For this review, take the finished solid that the model builds, in its own axes (mm). A direction names the side the tool comes from. Coordinates: 2 decimals unless noted, no trailing zeros. Order: outer loops, then holes, each group sorted by start corner. A loop starts at its lowest first (then second) coordinate and runs counter-clockwise, first axis right, second up. Notation, with made-up numbers: M 18,46.5 L 46,46.5 A21 cw 46,58.5 Z; hole C 60,11.5 d10. An arc over 180 degrees is marked long. Use one line per item in the form item = value. Start each with the question number.
```python
from build123d import *

# Parameters (mm, degrees)
SKETCH_1_W           = 200
SKETCH_1_H           = 250
EXTRUDE_1_DEPTH      = 5
CUT_EXTRUDE_1_DEPTH  = 35
CUT_EXTRUDE_2_DEPTH  = 35
CUT_EXTRUDE_5_DEPTH  = 30
CUT_EXTRUDE_6_DEPTH  = 10
SKETCH_9_R           = 1.5
CUT_EXTRUDE_8_DEPTH  = 10
SKETCH_10_R          = 1.5
CUT_EXTRUDE_9_DEPTH  = 10
CUT_EXTRUDE_12_DEPTH = 10
SKETCH_15_R          = 1.5
CUT_EXTRUDE_13_DEPTH = 10
SKETCH_16_R          = 1.5
CUT_EXTRUDE_14_DEPTH = 10
CUT_EXTRUDE_15_DEPTH = 10


with BuildPart() as part:
    # 草图1 → 凸台-拉伸1 (new body)
    with BuildSketch(Plane(origin=(0, 0, 0), x_dir=(1, 0, 0), z_dir=(0, 1, 0))):
        Rectangle(SKETCH_1_W, SKETCH_1_H)
    extrude(amount=EXTRUDE_1_DEPTH)

    # 草图2 → 切除-拉伸1 (cut)
    with BuildSketch(Plane(origin=(0, 5, 0), x_dir=(1, 0, 0), z_dir=(0, 1, 0))):
        Polygon((-100, -115), (-80, -125), (-100, -125), align=None)
    cut_extrude_1 = extrude(amount=-CUT_EXTRUDE_1_DEPTH, mode=Mode.SUBTRACT)

    # 镜向1: 切除-拉伸1 across plane
    add(cut_extrude_1.mirror(Plane(origin=(0, 0, 0), x_dir=(0, 0, 1), z_dir=(1, 0, 0))), mode=Mode.SUBTRACT)

    # 草图3 → 切除-拉伸2 (cut)
    with BuildSketch(Plane(origin=(0, 5, 0), x_dir=(1, 0, 0), z_dir=(0, 1, 0))):
        Polygon((-55, -125), (-50, -120), (0, -120), (0, -125), align=None)
    cut_extrude_2 = extrude(amount=-CUT_EXTRUDE_2_DEPTH, mode=Mode.SUBTRACT)

    # 镜向2: 切除-拉伸2 across plane
    add(cut_extrude_2.mirror(Plane(origin=(0, 0, 0), x_dir=(0, 0, 1), z_dir=(1, 0, 0))), mode=Mode.SUBTRACT)

    # 草图5 → 切除-拉伸5 (cut)
    with BuildSketch(Plane(origin=(0, 0, 0), x_dir=(1, 0, 0), z_dir=(0, 1, 0))):
        Polygon((-30, 125), (-100, 115), (-100, 125), align=None)
    cut_extrude_5 = extrude(amount=CUT_EXTRUDE_5_DEPTH, mode=Mode.SUBTRACT)

    # 镜向3: 切除-拉伸5 across plane
    add(cut_extrude_5.mirror(Plane(origin=(0, 0, 0), x_dir=(0, 0, 1), z_dir=(1, 0, 0))), mode=Mode.SUBTRACT)

    # 草图6 → 切除-拉伸6 (cut)
    with BuildSketch(Plane(origin=(0, 5, 0), x_dir=(1, 0, 0), z_dir=(0, 1, 0))):
        with BuildLine():
            Line((-100, 95), (-90, 95))
            Line((-90, 95), (-90, 105))
            Line((-90, 105), (-80, 105))
            ThreePointArc((-80, 105), (-75.121684822, 101.096376317), (-77.860612309, 95.480816412))
            Line((-77.860612309, 95.480816412), (-100, 85))
            Line((-100, 85), (-100, 95))
        make_face()
    cut_extrude_6 = extrude(amount=-CUT_EXTRUDE_6_DEPTH, mode=Mode.SUBTRACT)

    # 镜向4: 切除-拉伸6 across plane
    add(cut_extrude_6.mirror(Plane(origin=(0, 0, 0), x_dir=(0, 0, 1), z_dir=(1, 0, 0))), mode=Mode.SUBTRACT)

    # 草图9 → 切除-拉伸8 (cut)
    with BuildSketch(Plane(origin=(0, 5, 0), x_dir=(1, 0, 0), z_dir=(0, 1, 0))):
        with Locations((-80, -100)):
            Circle(SKETCH_9_R)
        with Locations((80, -100)):
            Circle(SKETCH_9_R)
    extrude(amount=-CUT_EXTRUDE_8_DEPTH, mode=Mode.SUBTRACT)

    # 草图10 → 切除-拉伸9 (cut)
    with BuildSketch(Plane(origin=(0, 5, 0), x_dir=(1, 0, 0), z_dir=(0, 1, 0))):
        with Locations((-80, 112.806380134)):
            Circle(SKETCH_10_R)
        with Locations((80, 112.806380134)):
            Circle(SKETCH_10_R)
    extrude(amount=-CUT_EXTRUDE_9_DEPTH, mode=Mode.SUBTRACT)

    # 草图14 → 切除-拉伸12 (cut)
    with BuildSketch(Plane(origin=(0, 5, 0), x_dir=(1, 0, 0), z_dir=(0, 1, 0))):
        with BuildLine():
            Line((-100, -85), (-72.5, -85))
            ThreePointArc((-72.5, -85), (-70.732233047, -84.267766953), (-70, -82.5))
            Line((-70, -82.5), (-70, -22.5))
            ThreePointArc((-70, -22.5), (-70.732233047, -20.732233047), (-72.5, -20))
            Line((-72.5, -20), (-100, -20))
            Line((-100, -20), (-100, -85))
        make_face()
        with BuildLine():
            Line((100, -20), (100, -85))
            Line((100, -85), (72.5, -85))
            ThreePointArc((72.5, -85), (70.732233047, -84.267766953), (70, -82.5))
            Line((70, -82.5), (70, -22.5))
            ThreePointArc((70, -22.5), (70.732233047, -20.732233047), (72.5, -20))
            Line((72.5, -20), (100, -20))
        make_face()
    extrude(amount=-CUT_EXTRUDE_12_DEPTH, mode=Mode.SUBTRACT)

    # 草图15 → 切除-拉伸13 (cut)
    with BuildSketch(Plane(origin=(0, 5, 0), x_dir=(1, 0, 0), z_dir=(0, 1, 0))):
        with Locations((-52.53096351, 0)):
            Circle(SKETCH_15_R)
        with Locations((-52.53096351, 86.645023586)):
            Circle(SKETCH_15_R)
        with Locations((52.53096351, 0)):
            Circle(SKETCH_15_R)
        with Locations((52.53096351, 86.645023586)):
            Circle(SKETCH_15_R)
    extrude(amount=-CUT_EXTRUDE_13_DEPTH, mode=Mode.SUBTRACT)

    # 草图16 → 切除-拉伸14 (cut)
    with BuildSketch(Plane.XZ):
        with Locations((60, 62.5)):
            Circle(SKETCH_16_R)
        with Locations((60, 42.5)):
            Circle(SKETCH_16_R)
        with Locations((36, 42.5)):
            Circle(SKETCH_16_R)
        with Locations((36, 62.5)):
            Circle(SKETCH_16_R)
    cut_extrude_14 = extrude(amount=-CUT_EXTRUDE_14_DEPTH, mode=Mode.SUBTRACT)

    # 镜向5: 切除-拉伸14 across plane
    add(cut_extrude_14.mirror(Plane(origin=(0, 0, 0), x_dir=(0, 0, 1), z_dir=(1, 0, 0))), mode=Mode.SUBTRACT)

    # 草图18 → 切除-拉伸15 (cut)
    with BuildSketch(Plane(origin=(0, 5, 0), x_dir=(1, 0, 0), z_dir=(0, 1, 0))):
        with BuildLine():
            Line((-19, -62.5), (19, -62.5))
            ThreePointArc((19, -62.5), (19.707106781, -62.207106781), (20, -61.5))
            Line((20, -61.5), (20, -43.5))
            ThreePointArc((20, -43.5), (19.707106781, -42.792893219), (19, -42.5))
            Line((19, -42.5), (-19, -42.5))
            ThreePointArc((-19, -42.5), (-19.707106781, -42.792893219), (-20, -43.5))
            Line((-20, -43.5), (-20, -61.5))
            ThreePointArc((-20, -61.5), (-19.707106781, -62.207106781), (-19, -62.5))
        make_face()
    extrude(amount=-CUT_EXTRUDE_15_DEPTH, mode=Mode.SUBTRACT)


solid = part.part
```
1. For pin 1 Ø2 at (x, z) = (-18, 45.5) entering from +Y; pin 2 Ø2.5 at (x, y) = (-94.5, 2.5) entering from +Z (3 decimals); pin 3 Ø2.5 at (y, z) = (2, 46) entering from -X; pin 4 Ø2.5 at (x, y) = (90, 1.5) entering from -Z, all flat-tipped, find the tip position at first contact; note any pin that passes through.
2. To check wall thickness, follow line 1 (Z direction, x = 88, y = 3.65); line 2 (Z direction, x = -13.5, y = 4.5); line 3 (Z direction, x = -79.5, y = 2.3). State the ranges of each line that lie inside material, in increasing order.
3. Consider section D-D, the plane x = -25. Write out the cut boundary in (y, z), plus the area to 4 significant figures.
4. Tool access review of faces 1 (the flat face through (1, 3, 120)), 2 (the flat face through (0, 3, 42.5)), 3 (the flat face through (-86, 3, 20)), 4 (the flat face through (-1, 5, -2)): name each direction out of +Z, -Z, +X, -X, +Y, -Y from which nothing blocks a thin tool from reaching the whole face with its end or side.
5. Consider section B-B, the plane x = 40.5. Write out the cut boundary in (y, z).
6. Consider section A-A, the plane x = -86. Write out the cut boundary in (y, z).
7. Consider section C-C, the plane y = 2.1. Give the number of separate pieces and of enclosed holes in the cut face, plus the area to 3 significant figures.
8. The part is to be moulded in two halves that separate along X. For faces 5 (the flat face through (-53, 3, 123)), 6 (the flat face through (90, 3, -100)), 7 (the flat face through (100, 2, 100)), 8 (the flat face through (-70, 3, 53)), say which applies: pulls with the +X half, pulls with the -X half, needs draft (parallel to the pull), parting line crosses it, or undercut.
Answers follow:
q1.pin_1 = through
q1.pin_2 = 118.375
q1.pin_3 = -70
q1.pin_4 = -116.61
q2.line_1 = -116.71 to -105, -90.68 to 20, 85 to 121
q2.line_2 = -125 to 42.5, 62.5 to 120
q2.line_3 = -117.93 to -114.22, -111.39 to -104.97, -94.7 to 20, 85 to 98.59, 101.41 to 125
q3.outline = M 0,-125 L 5,-125 L 5,120 L 0,120 Z
q3.area = 1,225 mm²
q4.face_1 = +Z, +Y, -Y
q4.face_2 = +Y, -Y
q4.face_3 = -X, +Y, -Y
q4.face_4 = +Z, -Z, +X, -X, +Y
q5.outline = M 0,-123.5 L 5,-123.5 L 5,120 L 0,120 Z
q6.outline = M 0,-117 L 5,-117 L 5,-105 L 0,-105 Z; M 0,-91.63 L 5,-91.63 L 5,20 L 0,20 Z; M 0,85 L 5,85 L 5,122 L 0,122 Z
q7.separate_pieces = 1
q7.enclosed_holes = 17
q7.area = 43,300 mm²
q8.face_5 = undercut
q8.face_6 = undercut
q8.face_7 = pulls with the +X half
q8.face_8 = pulls with the -X half
